Part print with two shaded views. Sizes in mm from the minimum x, y, z corner. A direction names the side the tool comes from. Round coordinates to 2 decimals unless told otherwise and drop trailing zeros. Write each loop counter-clockwise with the first axis right and the second up, starting at its lowest first coordinate (ties: lowest second). Pieces come first, ordered by that corner, then holes. Notation, with made-up numbers: M 86,29.5 L 97,29.5 A21 ccw 97,62.5 Z; hole C 44.5,-26 d6. An arc over 180 degrees is marked long. One line per question, with ' | ' between items. Start each with the question number.
1) Saw through at A-A (z = 4.5). List the corners of the cut face in (x, y) (1 decimal), plus the area to 3 significant figures.
2) Tool access for the marked faces 4 and 5: list every direction of +Z, -Z, +X, -X, +Y, -Y with a clear straight run to the whole face (end or side of a thin tool).
3) Mould opens along Y. For the marked faces 1, 2 and 3 say: pulls with the +Y half, pulls with the -Y half, needs draft (parallel to the pull), parting line crosses it, or undercut.
4) Wall check: probe 1 along X at (y, z) = (8, 2.15) (1 decimal); probe 2 along X at (y, z) = (10, 2.95) (1 decimal); probe 3 along Y at (x, z) = (26.5, 1.2). Give the ranges that are in metal, low to high. Write a range as [from, to].
5) Saw through at B-B (x = 44). List the corners of the cut face in (y, z) (1 decimal).
6) Saw through at C-C (y = 2.5). List the corners of the cut face in (x, z), plus the area to 3 significant figures.
7) Drop flat-ended pins along their axis: pin 1 Ø6 at (x, y) = (26.5, 3) entering from -Z; pin 2 Ø0.5 at (y, z) = (4, 3.5) entering from +X; pin 3 Ø1.8 at (y, z) = (9.5, 2) entering from +X (1 decimal); pin 4 Ø3 at (y, z) = (9.5, 1) entering from +X. Give the stop position or say it passes through.
8) Saw through at D-D (y = 6). List the corners of the cut face in (x, z) (1 decimal).
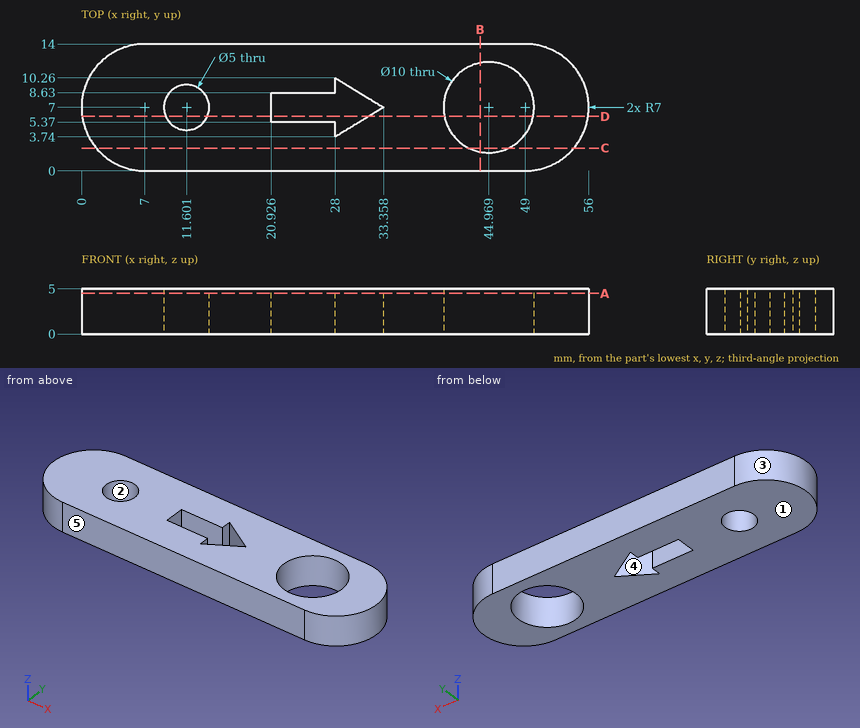
Answer key:
1) outline: M 7,0 L 49,0 A7 ccw 49,14 L 7,14 A7 ccw Z; hole C 11.6,7 d5; hole M 20.9,5.4 L 28,5.4 L 28,3.7 L 33.4,7 L 28,10.3 L 28,8.6 L 20.9,8.6 Z; hole C 45,7 d10 | area: 603 mm2
2) face 4: +Z, -Z | face 5: +Z, -Z, +X, -X, -Y
3) face 1: needs draft | face 2: undercut | face 3: parting line crosses it
4) probe 1: x = [0.1, 9.3], [13.9, 20.9], [31.7, 40.1], [49.9, 55.9] | probe 2: x = [0.7, 28], [28.4, 41], [49, 55.3] | probe 3: y = [0, 5.37], [8.63, 14]
5) outline: M 0,0 L 2.1,0 L 2.1,5 L 0,5 Z; M 11.9,0 L 14,0 L 14,5 L 11.9,5 Z
6) outline: M 1.64,0 L 42.79,0 L 42.79,5 L 1.64,5 Z; M 47.15,0 L 54.36,0 L 54.36,5 L 47.15,5 Z | area: 242 mm2
7) pin 1: stops at z = 0 | pin 2: stops at x = 55.44 | pin 3: stops at x = 55.8 | pin 4: stops at x = 55.93
8) outline: M 0.1,0 L 9.3,0 L 9.3,5 L 0.1,5 Z; M 13.9,0 L 20.9,0 L 20.9,5 L 13.9,5 Z; M 31.7,0 L 40.1,0 L 40.1,5 L 31.7,5 Z; M 49.9,0 L 55.9,0 L 55.9,5 L 49.9,5 Z
